```python
from build123d import *

# Parameters (mm, degrees)
F0_R     = 2
F1_DEPTH = 4
F2_R     = 2
F3_DEPTH = 4
F4_R     = 2
F5_DEPTH = 4
F6_R     = 10.310679
F7_DEPTH = 6.6
F8_SIZE  = 5


with BuildPart() as f1:
    # F0 (on Top) → F1 (new body)
    with BuildSketch(Plane.XY):
        Polygon((15, 50), (0, 50), (-4, 50), (-4, 0), (-4, -4), (50, -4), (50, 0), (50, 15), align=None)
        with Locations((26.219012, 7.5)):
            Circle(F0_R, mode=Mode.SUBTRACT)
        with Locations((41.652899, 7.5)):
            Circle(F0_R, mode=Mode.SUBTRACT)
        with Locations((7.5, 24.26653)):
            Circle(F0_R, mode=Mode.SUBTRACT)
        with Locations((7.5, 40.072314)):
            Circle(F0_R, mode=Mode.SUBTRACT)
    extrude(amount=F1_DEPTH)

    # F2 (on face) → F3 (join)
    with BuildSketch(Plane.XZ.offset(4)):
        Polygon((-4, 54), (-4, 4), (50, 4), (50, 19), (15, 54), align=None)
        with Locations((21.682408, 11.5)):
            Circle(F2_R, mode=Mode.SUBTRACT)
        with Locations((7.5, 24.480278)):
            Circle(F2_R, mode=Mode.SUBTRACT)
        with Locations((40.694896, 11.5)):
            Circle(F2_R, mode=Mode.SUBTRACT)
        with Locations((7.5, 42.723257)):
            Circle(F2_R, mode=Mode.SUBTRACT)
    extrude(amount=-F3_DEPTH)

    # F4 (on face) → F5 (join)
    with BuildSketch(Plane(origin=(-4, 0, 0), x_dir=(0, -1, 0), z_dir=(-1, 0, 0))):
        Polygon((-50, 0), (0, 0), (0, 54), (-15, 54), (-50, 19), align=None)
        with Locations((-38.723257, 11.5)):
            Circle(F4_R, mode=Mode.SUBTRACT)
        with Locations((-20.480278, 11.5)):
            Circle(F4_R, mode=Mode.SUBTRACT)
        with Locations((-7.5, 25.682408)):
            Circle(F4_R, mode=Mode.SUBTRACT)
        with Locations((-7.5, 44.694896)):
            Circle(F4_R, mode=Mode.SUBTRACT)
    extrude(amount=-F5_DEPTH)

    # F6 (on face) → F7 (join)
    with BuildSketch(Plane(origin=(0, 0, 0), x_dir=(1, 0, 0), z_dir=(0, 0, -1))):
        with Locations((23, -23)):
            Circle(F6_R)
    extrude(amount=F7_DEPTH)

    # F8
    f8_edges = [f1.edges().sort_by_distance(p)[0] for p in [
        (12.689321, 23, -6.6),
    ]]
    chamfer(f8_edges, length=F8_SIZE)


solid = f1.part
```
The listing builds one solid part. Answer for the finished solid, in the listing's coordinates (mm). A direction names the side the tool comes from. Give positions to 0.01 mm unless a question says otherwise; leave off trailing zeros. Loops run counter-clockwise (first coordinate to the right, second up) from the corner with the lowest first, then second, coordinate; pieces in that order, holes last. Notation, with made-up numbers: (52, 78.25) - (57, 78.25) arc R22 ccw to (57, 105.25) - close; hole circle Ø2 at (-8.75, 68). An arc over 180 degrees is marked (long way). Return JSON: item names as keys, results as strings. Group by question number.
1. Find section B-B (x = 7.5). Write down the section's boundary in (y, z).
2. Determine the mould class of faces 3 (the cylindrical face through (-2.028, 7.76, 46.678)), 4 (the flat face through (19, 20, 4)), 5 (the cylindrical face through (5.913, -2.028, 23.263)), 6 (the cylindrical face through (40.179, 8.852, 1.972)) for opening direction Z: pulls with the +Z half, pulls with the -Z half, needs draft (parallel to the pull), parting line crosses it, or undercut.
3. Find section D-D (x = 46.5). Write down the section's boundary in (y, z).
4. Given pin 1 Ø6.5 at (x, y) = (26.22, 7.5) entering from -Z; pin 2 Ø10 at (y, z) = (31.5, 36) entering from +X; pin 3 Ø6.5 at (x, z) = (40.69, 11.5) entering from +Y, each flat-ended and moving along its own axis, determine where each tip first touches the part or whether it passes through.
5. Which of the six approach directions +Z, -Z, +X, -X, +Y, -Y give full straight-line access (tool end or side, diameter ignored) to faces 1 (the flat face through (19, 0, 24)), 2 (the flat face through (-2, 32, 37))?
6. Straight lines are drawn through the part: line 1 (Z direction, x = 7.5, y = -1.15); line 2 (Y direction, x = 38, z = 10). For each, find the intervals that lie inside material, in ascending order. Write a range as [from, to].
7. Find section C-C (z = 48). Write down the section's boundary in (x, y).
8. Find section A-A (y = 7.5). Write down the section's boundary in (x, z), then the cut area to 3 significant figures.
Verdict:
{
 "1": {"outline": "(-4, 0) - (22.27, 0) - (22.27, 4) - (0, 4) - (0, 22.48) - (-4, 22.48) - close; (-4, 26.48) - (0, 26.48) - (0, 40.72) - (-4, 40.72) - close; (-4, 44.72) - (0, 44.72) - (0, 54) - (-4, 54) - close; (26.27, 0) - (38.07, 0) - (38.07, 4) - (26.27, 4) - close; (42.07, 0) - (50, 0) - (50, 4) - (42.07, 4) - close"},
 "2": {"face 3": "undercut", "face 4": "pulls with the +Z half", "face 5": "undercut", "face 6": "needs draft"},
 "3": {"outline": "(-4, 0) - (18.5, 0) - (18.5, 4) - (0, 4) - (0, 22.5) - (-4, 22.5) - close"},
 "4": {"pin 1": "stops at z = 0", "pin 2": "stops at x = 0", "pin 3": "stops at y = 0"},
 "5": {"face 1": "+Z, +X, +Y", "face 2": "+Z, +X, -X, +Y"},
 "6": {"line 1": "z = [0, 22.48], [26.48, 40.72], [44.72, 54]", "line 2": "y = [-4, 0]"},
 "7": {"outline": "(-4, -4) - (21, -4) - (21, 0) - (0, 0) - (0, 21) - (-4, 21) - close"},
 "8": {"outline": "(-4, 0) - (24.22, 0) - (24.22, 4) - (0, 4) - (0, 23.68) - (-4, 23.68) - close; (-4, 27.68) - (0, 27.68) - (0, 42.69) - (-4, 42.69) - close; (-4, 46.69) - (0, 46.69) - (0, 54) - (-4, 54) - close; (28.22, 0) - (39.65, 0) - (39.65, 4) - (28.22, 4) - close; (43.65, 0) - (50, 0) - (50, 4) - (43.65, 4) - close", "area": "352 mm^2"}
}
